from build123d import *

# Parameters (mm, degrees)
SKETCH_1_R          = 28.5
SKETCH_1_R_2        = 12.5
EXTRUDE_1_DEPTH     = 1.5
SKETCH_2_R          = 28.5
SKETCH_2_R_2        = 21.25
EXTRUDE_2_DEPTH     = 3
SKETCH_3_R          = 3
CUT_EXTRUDE_1_DEPTH = 1.5
SKETCH_4_R          = 1.6
CUT_EXTRUDE_2_DEPTH = 41.416580756


with BuildPart() as part:
    # 草图1 → 凸台-拉伸1 (new body)
    with BuildSketch(Plane(origin=(0, 0, 0), x_dir=(1, 0, 0), z_dir=(0, 1, 0))):
        with Locations(Location((0, 0, 0), (0, 0, 270))):
            Circle(SKETCH_1_R)
        with Locations(Location((0, 0, 0), (0, 0, 270))):
            Circle(SKETCH_1_R_2, mode=Mode.SUBTRACT)
    extrude(amount=EXTRUDE_1_DEPTH)

    # 草图2 → 凸台-拉伸2 (add)
    with BuildSketch(Plane(origin=(0, 1.5, 0), x_dir=(1, 0, 0), z_dir=(0, 1, 0))):
        with Locations(Location((0, 0, 0), (0, 0, 270))):
            Circle(SKETCH_2_R)
        with Locations(Location((0, 0, 0), (0, 0, 270))):
            Circle(SKETCH_2_R_2, mode=Mode.SUBTRACT)
    extrude(amount=EXTRUDE_2_DEPTH)

    # 草图3 → 切除-拉伸1 (cut)
    with BuildSketch(Plane(origin=(0, 4.5, 0), x_dir=(1, 0, 0), z_dir=(0, 1, 0))):
        with Locations(Location((0, 24.8, 0), (0, 0, 270))):
            Circle(SKETCH_3_R)
        with Locations(Location((24.8, 0, 0), (0, 0, 270))):
            Circle(SKETCH_3_R)
        with Locations(Location((0, -24.8, 0), (0, 0, 270))):
            Circle(SKETCH_3_R)
        with Locations(Location((-24.8, 0, 0), (0, 0, 270))):
            Circle(SKETCH_3_R)
    extrude(amount=-CUT_EXTRUDE_1_DEPTH, mode=Mode.SUBTRACT)

    # 草图4 → 切除-拉伸2 (cut, through all)
    with BuildSketch(Plane(origin=(0, 3, 0), x_dir=(1, 0, 0), z_dir=(0, 1, 0))):
        with Locations(Location((0, 24.8, 0), (0, 0, 270))):
            Circle(SKETCH_4_R)
        with Locations(Location((24.8, 0, 0), (0, 0, 270))):
            Circle(SKETCH_4_R)
        with Locations(Location((0, -24.8, 0), (0, 0, 270))):
            Circle(SKETCH_4_R)
        with Locations(Location((-24.8, 0, 0), (0, 0, 270))):
            Circle(SKETCH_4_R)
    extrude(amount=-CUT_EXTRUDE_2_DEPTH, mode=Mode.SUBTRACT)


solid = part.part
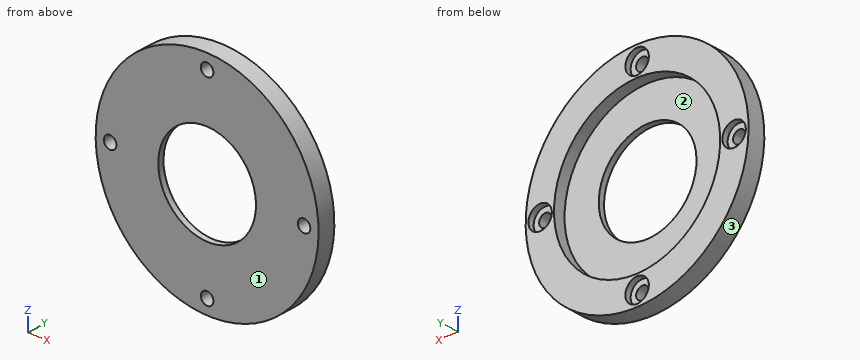
Geometry: final body of the model. Coordinates: model frame, mm. Face numbers are marked on the shaded views. Round coordinates to 2 decimals unless told otherwise and drop trailing zeros. Loops run counter-clockwise (first coordinate to the right, second up) from the corner with the lowest first, then second, coordinate; pieces in that order, holes last. Notation, with made-up numbers: M 0,5 L 44,5 A29 ccw 44,26 Z; hole C -6,-26.5 d6. An arc over 180 degrees is marked long. Put each result on its own line as item: value. Start each with the question number.
(1) Section query C-C (x = 15.5). Return loops of the section in (y, z).
(2) Contact query for flat-ended pins moving along their axis: pin 1 Ø1.8 at (x, z) = (24, -0.5) entering from +Y; pin 2 Ø1.5 at (x, y) = (9, 3) entering from +Z; pin 3 Ø2.5 at (x, z) = (0, -24.8) entering from +Y. Output: stop coordinate, or through.
(3) Section query A-A (x = -5). Return loops of the section in (y, z), then the cut area to 3 significant figures.
(4) Material intervals for line 1 along X through (y, z) = (2.2, 0); line 2 along X through (y, z) = (0.85, 0); line 3 along Y through (x, z) = (-6, -15), sorted ascending. Write a range as [from, to].
(5) Draft query along X for the marked faces 1, 2 and 3. Return one class per face: +X half, -X half, draft (parallel to the pull), parting line (faces both ways), or undercut.
(6) Section query D-D (z = 20.5). Return loops of the section in (x, y).
(7) Section query B-B (z = -6.5). Return loops of the section in (x, y), then the cut area to 3 significant figures.
Findings below:
1. outline: M 0,-23.92 L 4.5,-23.92 L 4.5,-14.54 L 1.5,-14.54 L 1.5,14.54 L 4.5,14.54 L 4.5,23.92 L 0,23.92 Z
2. pin 1: stops at y = 3
2. pin 2: stops at z = 27.28
2. pin 3: passes through
3. outline: M 0,-28.06 L 4.5,-28.06 L 4.5,-20.65 L 1.5,-20.65 L 1.5,-11.46 L 0,-11.46 Z; M 0,11.46 L 1.5,11.46 L 1.5,20.65 L 4.5,20.65 L 4.5,28.06 L 0,28.06 Z
3. area: 94.2 mm2
4. line 1: x = [-28.5, -26.4], [-23.2, -21.25], [21.25, 23.2], [26.4, 28.5]
4. line 2: x = [-28.5, -26.4], [-23.2, -12.5], [12.5, 23.2], [26.4, 28.5]
4. line 3: y = [0, 1.5]
5. face 1: draft
5. face 2: undercut
5. face 3: parting line
6. outline: M -19.8,0 L 19.8,0 L 19.8,4.5 L 5.6,4.5 L 5.6,1.5 L -5.6,1.5 L -5.6,4.5 L -19.8,4.5 Z
7. outline: M -27.75,0 L -10.68,0 L -10.68,1.5 L -20.23,1.5 L -20.23,4.5 L -27.75,4.5 Z; M 10.68,0 L 27.75,0 L 27.75,4.5 L 20.23,4.5 L 20.23,1.5 L 10.68,1.5 Z
7. area: 96.3 mm2
